from build123d import *

# Parameters (mm, degrees)
BOSS_EXTRUDE1_DEPTH = 3.175
SKETCH2_W           = 114.3
SKETCH2_H           = 3.175
CUT_EXTRUDE1_DEPTH  = 4.175


with BuildPart() as part:
    # Sketch1 → Boss-Extrude1 (new body)
    with BuildSketch(Plane(origin=(0, 0, 0), x_dir=(1, 0, 0), z_dir=(0, 1, 0))):
        Polygon((-42.852622222, 17.463911111), (109.547377778, 17.463911111), (109.547377778, 10.478911111), (106.372377778, 10.478911111), (106.372377778, 0.318911111), (109.547377778, 0.318911111), (109.547377778, -4.761088889), (106.372377778, -4.761088889), (106.372377778, -14.921088889), (109.547377778, -14.921088889), (109.547377778, -21.906088889), (-42.852622222, -21.906088889), (-42.852622222, -14.921088889), (-39.677622222, -14.921088889), (-39.677622222, -4.761088889), (-42.852622222, -4.761088889), (-42.852622222, 0.318911111), (-39.677622222, 0.318911111), (-39.677622222, 10.478911111), (-42.852622222, 10.478911111), align=None)
    extrude(amount=BOSS_EXTRUDE1_DEPTH)

    # Sketch2 → Cut-Extrude1 (cut, through all)
    with BuildSketch(Plane(origin=(0, 3.175, 0), x_dir=(1, 0, 0), z_dir=(0, 1, 0))):
        with Locations((33.347377778, -2.221088889)):
            Rectangle(SKETCH2_W, SKETCH2_H)
    extrude(amount=-CUT_EXTRUDE1_DEPTH, mode=Mode.SUBTRACT)


solid = part.part
Geometry check sheet. Reference: the model listing, model coordinates, mm. A direction names the side the tool comes from. Round coordinates to 2 decimals unless told otherwise and drop trailing zeros. Write each loop counter-clockwise with the first axis right and the second up, starting at its lowest first coordinate (ties: lowest second). Pieces come first, ordered by that corner, then holes. Notation, with made-up numbers: (61.25, 6) - (85.25, 6) arc R20 cw to (85.25, 23) - close; hole circle Ø7 at (38.25, 63). An arc over 180 degrees is marked (long way). One line per item, written item: value.
1. Scan lines: L1, parallel to X at y = 3.05, z = 1; L2, parallel to Z at x = 85, y = 0.2; L3, parallel to X at y = 2.8, z = -0.5. Record each from-to range of solid material in increasing order.
The answers:
L1: x = -42.85 to -23.8, 90.5 to 109.55
L2: z = -17.46 to 0.63, 3.81 to 21.91
L3: x = -39.68 to 106.37
2. Cross-section at C-C on z = 12. Record the boundary of the cut face in (x, y) (3 decimals), and give its area (3 significant figures).
The answers:
outline: (-39.678, 0) - (106.372, 0) - (106.372, 3.175) - (-39.678, 3.175) - close
area: 464 mm^2
3. Cross-section at B-B on y = 1.7. Record the boundary of the cut face in (x, z).
The answers:
outline: (-42.85, -17.46) - (109.55, -17.46) - (109.55, -10.48) - (106.37, -10.48) - (106.37, -0.32) - (109.55, -0.32) - (109.55, 4.76) - (106.37, 4.76) - (106.37, 14.92) - (109.55, 14.92) - (109.55, 21.91) - (-42.85, 21.91) - (-42.85, 14.92) - (-39.68, 14.92) - (-39.68, 4.76) - (-42.85, 4.76) - (-42.85, -0.32) - (-39.68, -0.32) - (-39.68, -10.48) - (-42.85, -10.48) - close; hole (-23.8, 0.63) - (90.5, 0.63) - (90.5, 3.81) - (-23.8, 3.81) - close
4. Depth check by flat-ended pin: pin 1 Ø3 at (x, z) = (10, 3.5) entering from +Y (3 decimals); pin 2 Ø1.6 at (y, z) = (2, 12) entering from -X; pin 3 Ø1 at (y, z) = (2, 12.5) entering from +X. Enter the tip coordinate at first touch or a pass-through.
The answers:
pin 1: stops at y = 3.175
pin 2: stops at x = -39.68
pin 3: stops at x = 106.37
5. Mould release check, pull along Z, two halves, no side actions. Record for faces 1 (the face through (108, 2, -10.479)), 2 (the face through (32, 2, -17.464)), 3 (the face through (-42.853, 2, 18)): released by +Z, released by -Z, zero draft, split by the parting line, or undercut.
The answers:
face 1: undercut
face 2: released by -Z
face 3: zero draft
6. Cross-section at A-A on x = 29. Record the boundary of the cut face in (y, z) (3 decimals).
The answers:
outline: (0, -17.464) - (3.175, -17.464) - (3.175, 0.634) - (0, 0.634) - close; (0, 3.809) - (3.175, 3.809) - (3.175, 21.906) - (0, 21.906) - close
7. Set-up check for faces 4 (the face through (106.372, 2, 10)), 5 (the face through (-39.678, 2, -5)), 6 (the face through (90.497, 2, 2)): record each of +Z, -Z, +X, -X, +Y, -Y from which the full face is reachable in a straight line by a thin tool's end or side.
The answers:
face 4: +X, +Y, -Y
face 5: -X, +Y, -Y
face 6: +Y, -Y
